Read the model definition and answer for the solid it produces. Units are mm, in the model's axes. A direction names the side the tool comes from. Give positions to 0.01 mm unless a question says otherwise; leave off trailing zeros. Order: outer loops, then holes, each group sorted by start corner. A loop starts at its lowest first (then second) coordinate and runs counter-clockwise, first axis right, second up. Notation, with made-up numbers: (-13, 62.25) -> (-6, 62.25) arc R23 cw to (-6, 79.25) -> close; hole circle Ø8 at (-27, -6.5). An arc over 180 degrees is marked (long way). Use one line per item in the form item = value.
```python
from build123d import *

# Parameters (mm, degrees)
SKETCH2_W          = 19.6
SKETCH2_H          = 19.6
CUT_EXTRUDE1_DEPTH = 1.5
CUT_EXTRUDE2_DEPTH = 5.2


with BuildPart() as part:
    # Sketch1 → Revolve1 (revolve)
    with BuildSketch(Plane(origin=(0, 0, 0), x_dir=(0, 0, -1), z_dir=(1, 0, 0))):
        with BuildLine():
            Line((-13.2, 0), (-13.2, 2.2845))
            Line((-13.2, 2.2845), (-12.767958406, 4.734729636))
            ThreePointArc((-12.767958406, 4.734729636), (-12.699554378, 4.853208889), (-12.570996856, 4.9))
            Line((-12.570996856, 4.9), (-11.7, 4.9))
            Line((-11.7, 4.9), (-11.7, 3.0595))
            ThreePointArc((-11.7, 3.0595), (-11.590165043, 2.794334957), (-11.325, 2.6845))
            Line((-11.325, 2.6845), (-10.8, 2.6845))
            Line((-10.8, 2.6845), (-10.8, 3.658578644))
            Line((-10.8, 3.658578644), (-10.658578644, 3.8))
            Line((-10.658578644, 3.8), (-10.4, 3.8))
            Line((-10.4, 3.8), (-10.4, 3.958043913))
            Line((-10.4, 3.958043913), (-9.8, 4))
            Line((-9.8, 4), (-0.6, 4))
            Line((-0.6, 4), (-0.5, 3.9))
            Line((-0.5, 3.9), (-0.4, 4))
            Line((-0.4, 4), (0, 4))
            Line((0, 4), (0, 2.5))
            Line((0, 2.5), (3.0095, 2.5))
            Line((3.0095, 2.5), (3.5, 2.0095))
            Line((3.5, 2.0095), (3.5, 0))
            Line((3.5, 0), (-13.2, 0))
        make_face()
    revolve(axis=Axis((0, 0, -3.5), (0, 0, 1)))

    # Sketch2 → Cut-Extrude1 (cut)
    with BuildSketch(Plane.XY.offset(13.2)):
        Rectangle(SKETCH2_W, SKETCH2_H)
        with BuildLine():
            Line((-3.9, 1), (-3.9, -1))
            ThreePointArc((-3.9, -1), (0, -4.9), (3.9, -1))
            Line((3.9, -1), (3.9, 1))
            ThreePointArc((3.9, 1), (0, 4.9), (-3.9, 1))
        make_face(mode=Mode.SUBTRACT)
    extrude(amount=-CUT_EXTRUDE1_DEPTH, mode=Mode.SUBTRACT)

    # Sketch3 → Cut-Extrude2 (cut)
    with BuildSketch(Plane.XY.offset(-3.5)):
        Polygon((-1.25, -0.721687836), (0, -1.443375673), (1.25, -0.721687836), (1.25, 0.721687836), (0, 1.443375673), (-1.25, 0.721687836), align=None)
    extrude(amount=CUT_EXTRUDE2_DEPTH, mode=Mode.SUBTRACT)

    # Sketch4 → Cut-Revolve1 (revolve, cut)
    with BuildSketch(Plane(origin=(0, 0, 0), x_dir=(0, 0, -1), z_dir=(1, 0, 0))):
        with BuildLine():
            Line((-13.2, 0), (-13.2, 2.2845))
            ThreePointArc((-13.2, 2.2845), (-13.112132034, 2.072367966), (-12.9, 1.9845))
            Line((-12.9, 1.9845), (-1.7, 1.9845))
            Line((-1.7, 1.9845), (-1.7, 0))
            Line((-1.7, 0), (-13.2, 0))
        make_face()
    revolve(axis=Axis((0, 0, 1.7), (0, 0, 1)), mode=Mode.SUBTRACT)


solid = part.part
```
Item 1: Given pin 1 Ø2 at (x, z) = (3, 10) entering from -Y; pin 2 Ø3 at (x, z) = (1.5, 2) entering from -Y; pin 3 Ø2 at (x, y) = (1.5, 3.5) entering from +Z, each flat-ended and moving along its own axis, determine where each tip first touches the part or whether it passes through.
Checks:
pin_1 = -3.45
pin_2 = -4
pin_3 = 13.11
Item 2: Which of the six approach directions +Z, -Z, +X, -X, +Y, -Y give full straight-line access (tool end or side, diameter ignored) to faces 1 (the cylindrical face through (3.905, -0.867, 0.197)), 2 (the cylindrical face through (-0.1, -4.9, 12.3)), 3 (the flat face through (-0.616, 1.088, -0.936))?
Checks:
face_1 = -Z
face_2 = +Z, -Z, -Y
face_3 = +Z, -Z
Item 3: Determine the mould class of faces 4 (the flat face through (-3, 0, 10.8)), 5 (the flat face through (1.25, 0, -1)), 6 (the cylindrical face through (-0.81, 2.56, 11.06)) for opening direction X: +X half, -X half, draft (parallel to the pull), parting line (faces both ways), or undercut.
Checks:
face_4 = draft
face_5 = undercut
face_6 = parting line
Item 4: Straight lines are drawn through the part: L1, parallel to X at y = 0, z = 4.75; L2, parallel to Z at x = 3.25, y = -1.5. For each, find the intervals that lie inside material, in ascending order. Write a range as from..to.
Checks:
L1 = -4..-1.98, 1.98..4
L2 = 0..10.8, 11.7..12.97
Item 5: The part is cut by section A-A on z = 2.75. Give the vertices of the cut face in (x, y).
Checks:
outline = circle Ø8 at (0, 0); hole circle Ø3.97 at (0, 0)
Item 6: The part is cut by section B-B on z = 10. Give the vertices of the cut face in (x, y), and give its area (3 significant figures).
Checks:
outline = circle Ø7.97 at (0, 0); hole circle Ø3.97 at (0, 0)
area = 37.5 mm²
